Geometry check sheet. Reference: the model listing, model coordinates, mm. A direction names the side the tool comes from. Give positions to 0.01 mm unless a question says otherwise; leave off trailing zeros. Loops run counter-clockwise (first coordinate to the right, second up) from the corner with the lowest first, then second, coordinate; pieces in that order, holes last.
1. Cross-section at A-A, the plane y = 34. Record the cut outline in (x, z).
2. Tool access check on faces 1 (the flat face through (-35.2, 51, -83)), 2 (the flat face through (-32, 34, -2)), 3 (the flat face through (33, 43, 1)). Record the directions out of +Z, -Z, +X, -X, +Y, -Y that give a thin tool (end or side, any length) a straight path to the whole face; none if there is none.
3. Go/stop test with flat-tipped pins: pin 1 Ø3 at (x, z) = (-10.5, -0.5) entering from +Y; pin 2 Ø3 at (x, y) = (22.91, 7.71) entering from +Z; pin 3 Ø5 at (x, y) = (22.91, 7.71) entering from -Z; pin 4 Ø3.5 at (y, z) = (51, 84) entering from +X. Record where each tip stops, or that it passes through.
4. Release check for a two-part mould opening along Z. For faces 4 (the flat face through (-35.2, 51, -33)), 5 (the cylindrical face through (22.673, 9.544, 107.535)) record: +Z half, -Z half, draft (parallel to the pull), parting line (faces both ways), or undercut.
5. Cross-section at B-B, the plane z = -54. Record the cut outline in (x, y), plus the area to 3 significant figures.
6. Material ranges on L1, parallel to X at y = 30, z = 65.5; L2, parallel to Z at x = 14, y = 35; L3, parallel to Y at x = -10, z = 1, recorded low to high.
Autodesk Inventor part; units mm, degrees
ref_plane "YZ Plane" through (0, 0, 0) normal (1, 0, 0) x (0, 1, 0)
ref_plane "XZ Plane" through (0, 0, 0) normal (0, 1, 0) x (-1, 0, 0)
ref_plane "XY Plane" through (0, 0, 0) normal (0, 0, 1) x (1, 0, 0)
sketch "Эскиз1" plane through (0, 0, 0) normal (0, 1, 0) x (-1, 0, 0)
  line L0 (-37, 110) -> (37, 110)
  line L1 (37, 110) -> (37, -110)
  line L2 (37, -110) -> (-37, -110)
  line L3 (-37, -110) -> (-37, 110)
  line L4 (-37, 110) -> (37, -110) construction
  line L5 (37, 110) -> (-37, -110) construction
  point P0 (0, 0)
  dimension "d0" = 74
  dimension "d1" = 220
extrude "Выдавливание1" add sketch "Эскиз1" along normal blind 43
sketch "Эскиз3" plane through (0, 43, 0) normal (0, 1, 0) x (1, 0, 0)
  line L0 (-32, -105) -> (32, -105)
  line L1 (32, -105) -> (32, 105)
  line L2 (32, 105) -> (-32, 105)
  line L3 (-32, 105) -> (-32, -105)
  line L4 (-32, -105) -> (32, 105) construction
  line L5 (32, -105) -> (-32, 105) construction
  line L6 (37, 110) -> (-37, 110)
  line L7 (-37, 110) -> (-37, -110)
  point P0 (0, 0)
  dimension "d4" = 5
  dimension "d5" = 5
extrude "Выдавливание2" cut sketch "Эскиз3" against normal blind 38
sketch "Эскиз4" plane through (0, 5, 0) normal (0, 1, 0) x (1, 0, 0)
  line L0 (32, 105) -> (32, -105)
  line L1 (32, 105) -> (0, 105)
  line L2 (0, 105) -> (0, 67.1211)
  line L3 (0, 67.1211) -> (32, 67.1211)
  line L4 (32, 67.1211) -> (32, 105)
  point P0 (0, 0)
sketch "Эскиз5" plane through (0, 43, 0) normal (0, 1, 0) x (1, 0, 0)
  line L0 (-37, 110) -> (-37, -110)
  line L1 (-37, -110) -> (37, -110)
  line L2 (-37, 110) -> (-32, 110)
  line L3 (-32, 110) -> (-32, -110)
  line L4 (-32, -110) -> (-37, -110)
  line L5 (-37, -110) -> (-37, 110)
  line L6 (-32, -105) -> (-32, 105)
  point P0 (0, 0)
  point P1 (-32, 0)
extrude "Выдавливание3" add sketch "Эскиз5" along normal blind 20
chamfer "Фаска1" distance 20 angle 45 2 edges at (-32, 43, -107.5) (-32, 43, 107.5)
sketch "Эскиз6" plane through (-37, 0, -110) normal (-1, 0, 0) x (0, 0, 1)
  circle A0 centre (25, 53) radius 2
  circle A1 centre (75, 53) radius 2
  line L0 (0, 63) -> (220, 63)
  point P0 (110, 0)
  dimension "d13" = 4
  dimension "d14" = 4
  dimension "d15" = 10
  dimension "d16" = 50
  dimension "d19" = 35
extrude "Выдавливание4" cut sketch "Эскиз6" against normal blind 10
mirror "Зеркальное отражение1" about plane through (0, 0, 0) normal (0, 0, 1) of "Выдавливание4"
sketch "Эскиз7" plane through (-37, 0, 110) normal (0, 0, 1) x (1, 0, 0)
  circle A0 centre (59.9136, 7.71) radius 1.85
  point P0 (37, 0)
extrude "Выдавливание5" cut sketch "Эскиз7" against normal through all
sketch "Эскиз8" plane through (-32, 5, 105) normal (1, 0, 0) x (0, 0, -1)
  circle A0 centre (20, 48) radius 2
  line L0 (20, 52.0415) -> (23.5, 50.0207)
  line L1 (23.5, 50.0207) -> (23.5, 45.9793)
  line L2 (23.5, 45.9793) -> (20, 43.9585)
  line L3 (20, 43.9585) -> (16.5, 45.9793)
  line L4 (16.5, 45.9793) -> (16.5, 50.0207)
  line L5 (16.5, 50.0207) -> (20, 52.0415)
  point P0 (105, -5)
  dimension "d22" = 7
extrude "Выдавливание6" cut sketch "Эскиз8" against normal blind 3.2 contours A0 | L0 L1 L2 L3 L4 L5
sketch "Эскиз9" plane through (-32, 5, 105) normal (1, 0, 0) x (0, 0, -1)
  circle A0 centre (70, 48) radius 2
  circle A1 centre (140, 48) radius 2
  circle A2 centre (190, 48) radius 2
  point P0 (105, -5)
pattern_sketch "Массив по эскизу1" of "Выдавливание6" from (-32, 53, 85) copies at (-32, 53, 35) at (-32, 53, -35) at (-32, 53, -85)
properties part number "KB33-046-008-001 - Корпус"
Result:
1. outline: (-37, -110) - (37, -110) - (37, 110) - (-37, 110) - close; hole (-32, -105) - (32, -105) - (32, 105) - (-32, 105) - close
2. face 1: +X
2. face 2: +Y
2. face 3: +Z, -Z, +X, +Y
3. pin 1: stops at y = 5
3. pin 2: passes through
3. pin 3: stops at z = -110
3. pin 4: stops at x = -32
4. face 4: undercut
4. face 5: draft
5. outline: (-37, 0) - (37, 0) - (37, 43) - (32, 43) - (32, 5) - (-32, 5) - (-32, 63) - (-37, 63) - close
5. area: 850 mm2
6. L1: x = -37 to -32, 32 to 37
6. L2: z = -110 to -105, 105 to 110
6. L3: y = 0 to 5
